from build123d import *

# Parameters (mm, degrees)
SKETCH1_W                                    = 101.6
SKETCH1_H                                    = 76.2
BOSS_EXTRUDE1_DEPTH                          = 50.8
CUT_EXTRUDE1_DEPTH                           = 31.75
CUT_EXTRUDE1_DEPTH_BACK                      = 31.75
SKETCH9_W                                    = 101.6
SKETCH9_H                                    = 41.275
F_45_64_0_70313_DIAMETER_HOLE1_D             = 17.859502
F_45_64_0_70313_DIAMETER_HOLE2_D             = 17.859502
F_45_64_0_70313_DIAMETER_HOLE2_DEPTH         = 25.4
F_45_64_0_70313_DIAMETER_HOLE2_TIP           = 5.365535714
CBORE_FOR_1_4_BINDING_HEAD_MACHINE_S_2_COUNT = 2
CBORE_FOR_1_4_BINDING_HEAD_MACHINE_S_2_PITCH = 22.098
CUT_EXTRUDE3_DEPTH                           = 137.783186101
F_8_32_TAPPED_HOLE1_D                        = 3.4544
F_8_32_TAPPED_HOLE1_DEPTH                    = 6.35


with BuildPart() as part:
    # Sketch1 → Boss-Extrude1 (new body)
    with BuildSketch(Plane(origin=(0, 0, 0), x_dir=(1, 0, 0), z_dir=(0, 1, 0))):
        with Locations((50.8, 38.1)):
            Rectangle(SKETCH1_W, SKETCH1_H)
    extrude(amount=BOSS_EXTRUDE1_DEPTH)

    # Sketch9 → Cut-Extrude1 (cut, two sides: drawn at the far end of the back side and taken through both)
    with BuildSketch(Plane.XY.offset(-38.1).offset(-CUT_EXTRUDE1_DEPTH_BACK)):
        with Locations((50.8, 30.1625)):
            Rectangle(SKETCH9_W, SKETCH9_H)
    extrude(amount=CUT_EXTRUDE1_DEPTH + CUT_EXTRUDE1_DEPTH_BACK, mode=Mode.SUBTRACT)

    # 45/64 (0.70313) Diameter Hole1 (through all)
    with Locations(Plane.XY):
        with Locations((50.8, 28.5242)):
            Hole(F_45_64_0_70313_DIAMETER_HOLE1_D / 2)

    # 45/64 (0.70313) Diameter Hole2
    with Locations(Plane.XY):
        with Locations((29.6418, 28.5242), (71.9582, 28.5242)):
            Hole(F_45_64_0_70313_DIAMETER_HOLE2_D / 2, depth=F_45_64_0_70313_DIAMETER_HOLE2_DEPTH)
            with Locations((0, 0, -(F_45_64_0_70313_DIAMETER_HOLE2_DEPTH + F_45_64_0_70313_DIAMETER_HOLE2_TIP / 2))):  # 118° drill point
                Cone(0, F_45_64_0_70313_DIAMETER_HOLE2_D / 2, F_45_64_0_70313_DIAMETER_HOLE2_TIP, mode=Mode.SUBTRACT)

    # Sketch14 → CBORE for 1/4 Binding Head Machine Screw1 (revolve, cut)
    with BuildSketch(Plane(origin=(50.8, 9.525, -50.8), x_dir=(0, 0, 1), z_dir=(1, 0, 0))):
        Polygon((0, 0), (0, 9.525), (3.3782, 9.525), (3.3782, 4.191), (7.14375, 4.191), (7.14375, 0.635), (7.77875, 0), align=None)
    cbore_for_1_4_binding_head_machine_screw = revolve(axis=Axis((50.8, 15.875, -50.8), (0, -1, 0)), mode=Mode.SUBTRACT)

    # CBORE for 1_4 Binding Head Machine S 2: CBORE for 1/4 Binding Head Machine Screw1 ×2
    with Locations(*[(0, 0, i * CBORE_FOR_1_4_BINDING_HEAD_MACHINE_S_2_PITCH) for i in range(1, CBORE_FOR_1_4_BINDING_HEAD_MACHINE_S_2_COUNT)]):
        add(cbore_for_1_4_binding_head_machine_screw, mode=Mode.SUBTRACT)

    # Sketch17 → Cut-Extrude3 (cut, through all)
    with BuildSketch(Plane.XY):
        Polygon((0, 25.4), (22.225, 47.625), (79.375, 47.625), (101.6, 25.4), (101.6, 50.8), (0, 50.8), align=None)
    extrude(amount=-CUT_EXTRUDE3_DEPTH, mode=Mode.SUBTRACT)

    # #8-32 Tapped Hole1
    with Locations(Plane(origin=(0, 0, -76.2), x_dir=(-1, 0, 0), z_dir=(0, 0, -1))):
        with Locations((-41.275, 38.0492), (-60.325, 18.9992), (-60.325, 38.0492), (-41.275, 18.9992)):
            Hole(F_8_32_TAPPED_HOLE1_D / 2, depth=F_8_32_TAPPED_HOLE1_DEPTH)


solid = part.part
Design review of the part built by this model. Coordinates are the model's own, in mm. A direction names the side the tool comes from. Coordinates: 2 decimals unless noted, no trailing zeros. Loops run counter-clockwise (first coordinate to the right, second up) from the corner with the lowest first, then second, coordinate; pieces in that order, holes last. Notation, with made-up numbers: M 76,82.25 L 89,82.25 A7 ccw 89,87.25 Z; hole C 31.5,18 d3. An arc over 180 degrees is marked long. Answer as CSV lines item,"result".
Item 1: The part is to be moulded in two halves that separate along Y. For faces 1 (the face through (11, 36.4, -73)), 2 (the face through (0, 7, -38)), 3 (the face through (39.904, 36.998, -72.981)), say which applies: pulls with the +Y half, pulls with the -Y half, needs draft (parallel to the pull), parting line crosses it, or undercut.
Answer list:
face 1,"pulls with the +Y half"
face 2,"needs draft"
face 3,"undercut"
Item 2: Machinability: for faces 4 (the face through (50, 16, -69.85)), 5 (the face through (36.223, 34.559, -3.219)), 6 (the face through (54, 5.334, -27)), 7 (the face through (58.6, 19.1, -73)), which of the approach directions +Z, -Z, +X, -X, +Y, -Y give a long, thin tool a straight path to every point of the face, cutting with its end or side? Answer none if there is none.
Answer list:
face 4,"+X, -X, +Y"
face 5,"+Z"
face 6,"+Y"
face 7,"-Z"
Item 3: Add section D-D on x = 29.5. State the section outline as (y, z) points (3 decimals), plus the area to 3 significant figures.
Answer list:
outline,"M 0,-76.2 L 47.625,-76.2 L 47.625,-69.85 L 9.525,-69.85 L 9.525,-6.35 L 19.596,-6.35 L 19.596,0 L 0,0 Z; M 37.453,-6.35 L 47.625,-6.35 L 47.625,0 L 37.453,0 Z"
area,"1,100 mm²"
Item 4: Add section A-A on z = -50.8. State the section outline as (x, y) points (3 decimals).
Answer list:
outline,"M 0,0 L 47.422,0 L 47.422,5.334 L 43.656,5.334 L 43.656,8.89 L 43.021,9.525 L 0,9.525 Z; M 54.178,0 L 101.6,0 L 101.6,9.525 L 58.579,9.525 L 57.944,8.89 L 57.944,5.334 L 54.178,5.334 Z"
Item 5: Add section C-C on x = 18. State the section outline as (y, z) points (3 decimals), plus the area to 3 significant figures.
Answer list:
outline,"M 0,-76.2 L 43.4,-76.2 L 43.4,-69.85 L 9.525,-69.85 L 9.525,-6.35 L 43.4,-6.35 L 43.4,0 L 0,0 Z"
area,"1,160 mm²"
Item 6: For P1, Ø3, axis at x = 41.28, y = 38.05, coming from the -Z side; P2, Ø7, axis at x = 48.5, z = -49.5, coming from the +Y side; P3, Ø11.5, axis at x = 51, z = -26, coming from the +Y side (3 decimals), all flat-tipped, find the tip position at first contact; note any pin that passes through.
Answer list:
P1,"z = -6.35"
P2,"y = 5.33"
P3,"y = 9.525"
Item 7: Add section B-B on y = 23.5. State the section outline as (x, z) points.
Answer list:
outline,"M 0,-76.2 L 43.42,-76.2 L 43.42,-69.85 L 0,-69.85 Z; M 0,-6.35 L 22.26,-6.35 L 22.26,0 L 0,0 Z; M 37.02,-6.35 L 43.42,-6.35 L 43.42,0 L 37.02,0 Z; M 58.18,-76.2 L 101.6,-76.2 L 101.6,-69.85 L 58.18,-69.85 Z; M 58.18,-6.35 L 64.58,-6.35 L 64.58,0 L 58.18,0 Z; M 79.34,-6.35 L 101.6,-6.35 L 101.6,0 L 79.34,0 Z"
Item 8: For probe 1 along Z at (x, y) = (50.8, 6); probe 2 along Z at (x, y) = (34, 44.5); probe 3 along Y at (x, z) = (68, -67.5) (3 decimals), list the stretches that pass through material, from the lowest coordinate up.
Answer list:
probe 1,"-76.2 to -57.94, -43.66 to -35.85, -21.56 to 0"
probe 2,"-76.2 to -69.85, -6.35 to 0"
probe 3,"0 to 9.525"
